Work out the finished part from the listing and answer in its coordinate system (mm). Face numbers are marked on the shaded views. A direction names the side the tool comes from. Round coordinates to 2 decimals unless told otherwise and drop trailing zeros. Loops run counter-clockwise (first coordinate to the right, second up) from the corner with the lowest first, then second, coordinate; pieces in that order, holes last. Notation, with made-up numbers: M 54,77 L 101,77 A24 cw 101,111 Z; hole C -11.5,46 d4. An arc over 180 degrees is marked long. One line per item, written item: value.
```python
from build123d import *

# Parameters (mm, degrees)
SKETCH1_W           = 54
SKETCH1_H           = 46
SKETCH1_W_2         = 48
SKETCH1_H_2         = 40
BOSS_EXTRUDE1_DEPTH = 50
SKETCH2_W           = 54
SKETCH2_H           = 10
SKETCH2_R           = 1.65
SKETCH2_W_2         = 13
SKETCH2_H_2         = 14
BOSS_EXTRUDE2_DEPTH = 5


with BuildPart() as part:
    # Sketch1 → Boss-Extrude1 (new body)
    with BuildSketch(Plane(origin=(0, 0, 0), x_dir=(1, 0, 0), z_dir=(0, 1, 0))):
        with Locations((2.264566872, 0.439206794)):
            Rectangle(SKETCH1_W, SKETCH1_H)
        with Locations((2.264566872, 0.439206794)):
            Rectangle(SKETCH1_W_2, SKETCH1_H_2, mode=Mode.SUBTRACT)
    extrude(amount=BOSS_EXTRUDE1_DEPTH)

    # Sketch2 → Boss-Extrude2 (add)
    # profile 1 of 2: a face of its own
    with BuildSketch(Plane(origin=(0, 0, 0), x_dir=(1, 0, 0), z_dir=(0, 1, 0))):
        with Locations((2.264566872, 28.439206794)):
            Rectangle(SKETCH2_W, SKETCH2_H)
        with Locations(Location((-18.235433128, 28.439206794, 0), (0, 0, 270))):
            Circle(SKETCH2_R, mode=Mode.SUBTRACT)
        with Locations(Location((1.764566872, 28.439206794, 0), (0, 0, 270))):
            Circle(SKETCH2_R, mode=Mode.SUBTRACT)
        with Locations(Location((21.764566872, 28.439206794, 0), (0, 0, 270))):
            Circle(SKETCH2_R, mode=Mode.SUBTRACT)
    # profile 2 of 2: a face of its own
    with BuildSketch(Plane(origin=(0, 0, 0), x_dir=(1, 0, 0), z_dir=(0, 1, 0))):
        with Locations((-18.235433128, -29.560793206)):
            Rectangle(SKETCH2_W_2, SKETCH2_H_2)
        with Locations(Location((-18.235433128, -31.560793206, 0), (0, 0, 270))):
            Circle(SKETCH2_R, mode=Mode.SUBTRACT)
    extrude(amount=BOSS_EXTRUDE2_DEPTH)


solid = part.part
```
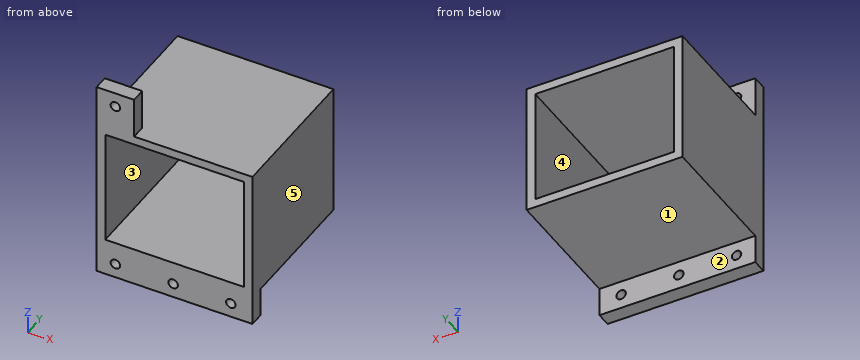
1) Find section A-A (x = -13). Give the vertices of the cut face in (y, z).
Check values:
outline: M 0,-33.44 L 5,-33.44 L 5,-23.44 L 50,-23.44 L 50,-20.44 L 0,-20.44 Z; M 0,19.56 L 50,19.56 L 50,22.56 L 5,22.56 L 5,36.56 L 0,36.56 Z
2) Find section B-B (z = -18.5). Give the vertices of the cut face in (x, y).
Check values:
outline: M -24.74,0 L -21.74,0 L -21.74,50 L -24.74,50 Z; M 26.26,0 L 29.26,0 L 29.26,50 L 26.26,50 Z
3) For the marked faces 4 and 5, determine the directions among +Z, -Z, +X, -X, +Y, -Y from which every point of the face is accessible in a straight line to the end or side of a thin tool.
Check values:
face 4: +Y, -Y
face 5: +Z, -Z, +X, +Y, -Y
4) Each of these flat-tipped pins is pushed along its axis until it touches: pin 1 (2.5 mm diameter, centred on y = 2, z = 26.5, fed in from +X); pin 2 (3 mm diameter, centred on x = 11.5, z = -28.5, fed in from +Y); pin 3 (5 mm diameter, centred on x = -18, y = 36.5, fed in from -Z); pin 4 (3 mm diameter, centred on x = 21.76, z = -28.44, fed in from -Y). Where does it stop, or does it pass through?
Check values:
pin 1: x = -11.74
pin 2: y = 5
pin 3: z = -23.44
pin 4: through
5) Find section D-D (y = 4). Give the vertices of the cut face in (x, z).
Check values:
outline: M -24.74,-33.44 L 29.26,-33.44 L 29.26,22.56 L -11.74,22.56 L -11.74,36.56 L -24.74,36.56 Z; hole M -21.74,-20.44 L 26.26,-20.44 L 26.26,19.56 L -21.74,19.56 Z; hole C -18.24,-28.44 d3.3; hole C -18.24,31.56 d3.3; hole C 1.76,-28.44 d3.3; hole C 21.76,-28.44 d3.3
6) The mould has two halves that part along Z. Classify the marked faces 1, 2 and 3: +Z half, -Z half, draft (parallel to the pull), parting line (faces both ways), or undercut.
Check values:
face 1: -Z half
face 2: draft
face 3: undercut
7) Find the intervals of material crossed by probe 1 along Z at (x, y) = (24.5, 3); probe 2 along Z at (x, y) = (24, 10.5); probe 3 along X at (y, z) = (41, -11), in increasing order. Write a range as from..to.
Check values:
probe 1: -33.44..-20.44, 19.56..22.56
probe 2: -23.44..-20.44, 19.56..22.56
probe 3: -24.74..-21.74, 26.26..29.26
8) Find section C-C (y = 32). Give the vertices of the cut face in (x, z).
Check values:
outline: M -24.74,-23.44 L 29.26,-23.44 L 29.26,22.56 L -24.74,22.56 Z; hole M -21.74,-20.44 L 26.26,-20.44 L 26.26,19.56 L -21.74,19.56 Z
